```python
from build123d import *

# Parameters (mm, degrees)
BOSS_EXTRUDE1_DEPTH = 26.5
SKETCH3_R           = 10.9
CUT_EXTRUDE1_DEPTH  = 129.322835068
SKETCH6_W           = 26.5
SKETCH6_H           = 26.5
BOSS_EXTRUDE3_DEPTH = 80
SKETCH7_R           = 10.9
CUT_EXTRUDE2_DEPTH  = 200.766738973
FILLET1_R           = 10


with BuildPart() as part:
    # Sketch2 → Boss-Extrude1 (new body)
    with BuildSketch(Plane(origin=(0, 0, 0), x_dir=(1, 0, 0), z_dir=(0, 1, 0))):
        Polygon((0, 0), (0, 66.5), (106.5, 66.5), (106.5, 40), (26.5, 40), (26.5, 0), align=None)
    extrude(amount=BOSS_EXTRUDE1_DEPTH)

    # Sketch3 → Cut-Extrude1 (cut, through all)
    with BuildSketch(Plane.XY):
        with Locations((13.25, 13.25)):
            Circle(SKETCH3_R)
    extrude(amount=-CUT_EXTRUDE1_DEPTH, mode=Mode.SUBTRACT)

    # Sketch6 → Boss-Extrude3 (add)
    with BuildSketch(Plane.ZY):
        with Locations((-53.25, 13.25)):
            Rectangle(SKETCH6_W, SKETCH6_H)
    extrude(amount=BOSS_EXTRUDE3_DEPTH)

    # Sketch7 → Cut-Extrude2 (cut, through all)
    with BuildSketch(Plane.ZY.offset(80)):
        with Locations((-53.25, 13.25)):
            Circle(SKETCH7_R)
    extrude(amount=-CUT_EXTRUDE2_DEPTH, mode=Mode.SUBTRACT)

    # Fillet1
    # the kernel refuses this fillet: 10 mm, written as the material it takes off along each edge
    with BuildSketch(Plane(origin=(106.5, 26.5, -40), x_dir=(0, 0, -1), z_dir=(-1, 0, 0))) as fillet1_piece_1:
        with BuildLine():
            CenterArc((FILLET1_R, FILLET1_R), FILLET1_R, 180, 90)
            Line((0, FILLET1_R), (-FILLET1_R * 0.02, FILLET1_R))
            Line((-FILLET1_R * 0.02, FILLET1_R), (-FILLET1_R * 0.02, -FILLET1_R * 0.02))
            Line((-FILLET1_R * 0.02, -FILLET1_R * 0.02), (FILLET1_R, -FILLET1_R * 0.02))
            Line((FILLET1_R, -FILLET1_R * 0.02), (FILLET1_R, 0))
        make_face()
    extrude(amount=80, mode=Mode.SUBTRACT)
    with BuildSketch(Plane(origin=(106.5, 26.5, -66.5), x_dir=(0, 0, 1), z_dir=(-1, 0, 0)), Plane(origin=(-80, 0, -66.5), x_dir=(0, 0, 1), z_dir=(1, 0, 0))) as fillet1_piece_2:
        with BuildLine():
            CenterArc((FILLET1_R, -FILLET1_R), FILLET1_R, 90, 90)
            Line((0, -FILLET1_R), (-FILLET1_R * 0.02, -FILLET1_R))
            Line((-FILLET1_R * 0.02, -FILLET1_R), (-FILLET1_R * 0.02, FILLET1_R * 0.02))
            Line((-FILLET1_R * 0.02, FILLET1_R * 0.02), (FILLET1_R, FILLET1_R * 0.02))
            Line((FILLET1_R, FILLET1_R * 0.02), (FILLET1_R, 0))
        make_face()
    extrude(amount=186.5, mode=Mode.SUBTRACT)
    with BuildSketch(Plane(origin=(0, 0, 0), x_dir=(0, 1, 0), z_dir=(0, 0, -1)), Plane(origin=(26.5, 26.5, -40), x_dir=(-1, 0, 0), z_dir=(0, 0, 1))) as fillet1_piece_3:
        with BuildLine():
            CenterArc((FILLET1_R, FILLET1_R), FILLET1_R, 180, 90)
            Line((0, FILLET1_R), (-FILLET1_R * 0.02, FILLET1_R))
            Line((-FILLET1_R * 0.02, FILLET1_R), (-FILLET1_R * 0.02, -FILLET1_R * 0.02))
            Line((-FILLET1_R * 0.02, -FILLET1_R * 0.02), (FILLET1_R, -FILLET1_R * 0.02))
            Line((FILLET1_R, -FILLET1_R * 0.02), (FILLET1_R, 0))
        make_face()
    extrude(amount=40, mode=Mode.SUBTRACT)
    with BuildSketch(Plane(origin=(0, 26.5, 0), x_dir=(0, -1, 0), z_dir=(0, 0, -1)), Plane(origin=(26.5, 0, -40), x_dir=(-1, 0, 0), z_dir=(0, 0, 1))) as fillet1_piece_4:
        with BuildLine():
            CenterArc((FILLET1_R, -FILLET1_R), FILLET1_R, 90, 90)
            Line((0, -FILLET1_R), (-FILLET1_R * 0.02, -FILLET1_R))
            Line((-FILLET1_R * 0.02, -FILLET1_R), (-FILLET1_R * 0.02, FILLET1_R * 0.02))
            Line((-FILLET1_R * 0.02, FILLET1_R * 0.02), (FILLET1_R, FILLET1_R * 0.02))
            Line((FILLET1_R, FILLET1_R * 0.02), (FILLET1_R, 0))
        make_face()
    extrude(amount=40, mode=Mode.SUBTRACT)
    with BuildSketch(Plane(origin=(0, 0, -40), x_dir=(0, 0, -1), z_dir=(-1, 0, 0)), Plane(origin=(0, 26.5, -40), x_dir=(0, -1, 0), z_dir=(-1, 0, 0)), Plane(origin=(106.5, 0, -40), x_dir=(0, 0, -1), z_dir=(-1, 0, 0))) as fillet1_piece_5:
        with BuildLine():
            CenterArc((FILLET1_R, -FILLET1_R), FILLET1_R, 90, 90)
            Line((0, -FILLET1_R), (-FILLET1_R * 0.02, -FILLET1_R))
            Line((-FILLET1_R * 0.02, -FILLET1_R), (-FILLET1_R * 0.02, FILLET1_R * 0.02))
            Line((-FILLET1_R * 0.02, FILLET1_R * 0.02), (FILLET1_R, FILLET1_R * 0.02))
            Line((FILLET1_R, FILLET1_R * 0.02), (FILLET1_R, 0))
        make_face()
    extrude(amount=80, mode=Mode.SUBTRACT)
    with BuildSketch(Plane(origin=(106.5, 26.5, -40), x_dir=(0, 0, -1), z_dir=(-1, 0, 0))) as fillet1_piece_6a_section:
        with BuildLine():
            CenterArc((FILLET1_R, FILLET1_R), FILLET1_R, 180, 90)
            Line((0, FILLET1_R), (-FILLET1_R * 0.02, FILLET1_R))
            Line((-FILLET1_R * 0.02, FILLET1_R), (-FILLET1_R * 0.02, -FILLET1_R * 0.02))
            Line((-FILLET1_R * 0.02, -FILLET1_R * 0.02), (FILLET1_R, -FILLET1_R * 0.02))
            Line((FILLET1_R, -FILLET1_R * 0.02), (FILLET1_R, 0))
        make_face()
    fillet1_piece_6a = extrude(amount=105, mode=Mode.PRIVATE)
    fillet1_piece_6a = split(fillet1_piece_6a, bisect_by=Plane(origin=(26.5, 24.236048857, -42.263951143), z_dir=(-1, 0, 0)), keep=Keep.TOP, mode=Mode.PRIVATE)
    with BuildSketch(Plane(origin=(26.5, 26.5, -65), x_dir=(-1, 0, 0), z_dir=(0, 0, 1))) as fillet1_piece_6b_section:
        with BuildLine():
            CenterArc((FILLET1_R, FILLET1_R), FILLET1_R, 180, 90)
            Line((0, FILLET1_R), (-FILLET1_R * 0.02, FILLET1_R))
            Line((-FILLET1_R * 0.02, FILLET1_R), (-FILLET1_R * 0.02, -FILLET1_R * 0.02))
            Line((-FILLET1_R * 0.02, -FILLET1_R * 0.02), (FILLET1_R, -FILLET1_R * 0.02))
            Line((FILLET1_R, -FILLET1_R * 0.02), (FILLET1_R, 0))
        make_face()
    fillet1_piece_6b = extrude(amount=65, mode=Mode.PRIVATE)
    fillet1_piece_6b = split(fillet1_piece_6b, bisect_by=Plane(origin=(24.236048857, 24.236048857, -40), z_dir=(0, 0, -1)), keep=Keep.TOP, mode=Mode.PRIVATE)
    fillet1_piece_6 = fillet1_piece_6a & fillet1_piece_6b
    add(fillet1_piece_6, mode=Mode.SUBTRACT)
    with BuildSketch(Plane(origin=(0, 0, 0), x_dir=(0, 1, 0), z_dir=(0, 0, -1))) as fillet1_piece_7a_section:
        with BuildLine():
            CenterArc((FILLET1_R, FILLET1_R), FILLET1_R, 180, 90)
            Line((0, FILLET1_R), (-FILLET1_R * 0.02, FILLET1_R))
            Line((-FILLET1_R * 0.02, FILLET1_R), (-FILLET1_R * 0.02, -FILLET1_R * 0.02))
            Line((-FILLET1_R * 0.02, -FILLET1_R * 0.02), (FILLET1_R, -FILLET1_R * 0.02))
            Line((FILLET1_R, -FILLET1_R * 0.02), (FILLET1_R, 0))
        make_face()
    fillet1_piece_7a = extrude(amount=65, mode=Mode.PRIVATE)
    fillet1_piece_7a = split(fillet1_piece_7a, bisect_by=Plane(origin=(2.263951143, 2.263951143, -40), z_dir=(0, 0, -1)), keep=Keep.TOP, mode=Mode.PRIVATE)
    with BuildSketch(Plane(origin=(25, 0, -40), x_dir=(0, 0, -1), z_dir=(-1, 0, 0))) as fillet1_piece_7b_section:
        with BuildLine():
            CenterArc((FILLET1_R, -FILLET1_R), FILLET1_R, 90, 90)
            Line((0, -FILLET1_R), (-FILLET1_R * 0.02, -FILLET1_R))
            Line((-FILLET1_R * 0.02, -FILLET1_R), (-FILLET1_R * 0.02, FILLET1_R * 0.02))
            Line((-FILLET1_R * 0.02, FILLET1_R * 0.02), (FILLET1_R, FILLET1_R * 0.02))
            Line((FILLET1_R, FILLET1_R * 0.02), (FILLET1_R, 0))
        make_face()
    fillet1_piece_7b = extrude(amount=105, mode=Mode.PRIVATE)
    fillet1_piece_7b = split(fillet1_piece_7b, bisect_by=Plane(origin=(0, 2.263951143, -42.263951143), z_dir=(1, 0, 0)), keep=Keep.TOP, mode=Mode.PRIVATE)
    fillet1_piece_7 = fillet1_piece_7a & fillet1_piece_7b
    add(fillet1_piece_7, mode=Mode.SUBTRACT)
    with BuildSketch(Plane(origin=(0, 26.5, 0), x_dir=(0, -1, 0), z_dir=(0, 0, -1))) as fillet1_piece_8a_section:
        with BuildLine():
            CenterArc((FILLET1_R, -FILLET1_R), FILLET1_R, 90, 90)
            Line((0, -FILLET1_R), (-FILLET1_R * 0.02, -FILLET1_R))
            Line((-FILLET1_R * 0.02, -FILLET1_R), (-FILLET1_R * 0.02, FILLET1_R * 0.02))
            Line((-FILLET1_R * 0.02, FILLET1_R * 0.02), (FILLET1_R, FILLET1_R * 0.02))
            Line((FILLET1_R, FILLET1_R * 0.02), (FILLET1_R, 0))
        make_face()
    fillet1_piece_8a = extrude(amount=65, mode=Mode.PRIVATE)
    fillet1_piece_8a = split(fillet1_piece_8a, bisect_by=Plane(origin=(2.263951143, 24.236048857, -40), z_dir=(0, 0, -1)), keep=Keep.TOP, mode=Mode.PRIVATE)
    with BuildSketch(Plane(origin=(25, 26.5, -40), x_dir=(0, -1, 0), z_dir=(-1, 0, 0))) as fillet1_piece_8b_section:
        with BuildLine():
            CenterArc((FILLET1_R, -FILLET1_R), FILLET1_R, 90, 90)
            Line((0, -FILLET1_R), (-FILLET1_R * 0.02, -FILLET1_R))
            Line((-FILLET1_R * 0.02, -FILLET1_R), (-FILLET1_R * 0.02, FILLET1_R * 0.02))
            Line((-FILLET1_R * 0.02, FILLET1_R * 0.02), (FILLET1_R, FILLET1_R * 0.02))
            Line((FILLET1_R, FILLET1_R * 0.02), (FILLET1_R, 0))
        make_face()
    fillet1_piece_8b = extrude(amount=105, mode=Mode.PRIVATE)
    fillet1_piece_8b = split(fillet1_piece_8b, bisect_by=Plane(origin=(0, 24.236048857, -42.263951143), z_dir=(1, 0, 0)), keep=Keep.TOP, mode=Mode.PRIVATE)
    fillet1_piece_8 = fillet1_piece_8a & fillet1_piece_8b
    add(fillet1_piece_8, mode=Mode.SUBTRACT)
    with BuildSketch(Plane(origin=(106.5, 0, -40), x_dir=(0, 0, -1), z_dir=(-1, 0, 0))) as fillet1_piece_9a_section:
        with BuildLine():
            CenterArc((FILLET1_R, -FILLET1_R), FILLET1_R, 90, 90)
            Line((0, -FILLET1_R), (-FILLET1_R * 0.02, -FILLET1_R))
            Line((-FILLET1_R * 0.02, -FILLET1_R), (-FILLET1_R * 0.02, FILLET1_R * 0.02))
            Line((-FILLET1_R * 0.02, FILLET1_R * 0.02), (FILLET1_R, FILLET1_R * 0.02))
            Line((FILLET1_R, FILLET1_R * 0.02), (FILLET1_R, 0))
        make_face()
    fillet1_piece_9a = extrude(amount=105, mode=Mode.PRIVATE)
    fillet1_piece_9a = split(fillet1_piece_9a, bisect_by=Plane(origin=(26.5, 2.263951143, -42.263951143), z_dir=(-1, 0, 0)), keep=Keep.TOP, mode=Mode.PRIVATE)
    with BuildSketch(Plane(origin=(26.5, 0, -65), x_dir=(-1, 0, 0), z_dir=(0, 0, 1))) as fillet1_piece_9b_section:
        with BuildLine():
            CenterArc((FILLET1_R, -FILLET1_R), FILLET1_R, 90, 90)
            Line((0, -FILLET1_R), (-FILLET1_R * 0.02, -FILLET1_R))
            Line((-FILLET1_R * 0.02, -FILLET1_R), (-FILLET1_R * 0.02, FILLET1_R * 0.02))
            Line((-FILLET1_R * 0.02, FILLET1_R * 0.02), (FILLET1_R, FILLET1_R * 0.02))
            Line((FILLET1_R, FILLET1_R * 0.02), (FILLET1_R, 0))
        make_face()
    fillet1_piece_9b = extrude(amount=65, mode=Mode.PRIVATE)
    fillet1_piece_9b = split(fillet1_piece_9b, bisect_by=Plane(origin=(24.236048857, 2.263951143, -40), z_dir=(0, 0, -1)), keep=Keep.TOP, mode=Mode.PRIVATE)
    fillet1_piece_9 = fillet1_piece_9a & fillet1_piece_9b
    add(fillet1_piece_9, mode=Mode.SUBTRACT)


solid = part.part
```
The listing builds one solid part. Answer for the finished solid, in the listing's coordinates (mm). A direction names the side the tool comes from. Round coordinates to 2 decimals unless told otherwise and drop trailing zeros. Loops run counter-clockwise (first coordinate to the right, second up) from the corner with the lowest first, then second, coordinate; pieces in that order, holes last. Notation, with made-up numbers: (5, 50) - (41, 50) arc R12 cw to (41, 64) - close; hole circle Ø7 at (14.25, 36.5). An arc over 180 degrees is marked (long way). Use one line per item in the form item = value. Start each with the question number.
1. Consider line 1 (Y direction, x = -18, z = -53.25); line 2 (Z direction, x = 84, y = 13.25). Determine where each line is inside the solid, lowest interval first. Write a range as [from, to].
2. The part is cut by section A-A on y = 13.25. Determine the outline of the cut face in (x, z).
3. For a pull along Y with two mould halves and no side action, classify faces 5 (the face through (0, 13, -20)), 6 (the face through (-34.03, 2.61, -55.61)), 7 (the face through (14, 0, -47)) as pulls with the +Y half, pulls with the -Y half, needs draft (parallel to the pull), parting line crosses it, or undercut.
4. Given pin 1 Ø8 at (y, z) = (20, -16.5) entering from +X; pin 2 Ø2 at (y, z) = (14, -13) entering from -X; pin 3 Ø12 at (x, z) = (37.5, -39) entering from -Y, each flat-ended and moving along its own axis, determine where each tip first touches the part or whether it passes through.
5. The part is cut by section C-C on z = -36.5. Determine the outline of the cut face in (x, y), then the cut area to 3 significant figures.
6. A tool of negligible diameter and unlimited length cuts with its end or side. For faces 1 (the face through (-34.37, 2.85, -43.01)), 2 (the face through (26.5, 13, -20)), 3 (the face through (23.65, 23.49, -19.79)), 4 (the face through (-34.37, 23.49, -42.85)), from which of +Z, -Z, +X, -X, +Y, -Y can it reach the whole face along a straight path? Write none if from no direction.
7. The part is cut by section D-D on z = -48. Determine the outline of the cut face in (x, y).
8. The part is cut by section B-B on x = 89.5. Determine the outline of the cut face in (y, z), then the cut area to 3 significant figures.
Geometry check:
q1.line_1 = [0, 2.35], [24.15, 26.5]
q1.line_2 = [-66.5, -64.15], [-42.35, -40]
q2.outline = (-80, -66.5) - (2.35, -66.5) - (2.35, -64.15) - (-80, -64.15) - close; (-80, -42.35) - (2.35, -42.35) - (2.35, 0) - (0, 0) - (0, -40) - (-80, -40) - close; (24.15, -66.5) - (106.5, -66.5) - (106.5, -64.15) - (24.15, -64.15) - close; (24.15, -42.35) - (106.5, -42.35) - (106.5, -40) - (26.5, -40) - (26.5, 0) - (24.15, 0) - close
q3.face_5 = needs draft
q3.face_6 = undercut
q3.face_7 = pulls with the -Y half
q4.pin_1 = 26.5
q4.pin_2 = 0
q4.pin_3 = 1.34
q5.outline = (0, 10) arc R10 ccw to (10, 0) - (16.5, 0) arc R10 ccw to (26.5, 10) - (26.5, 16.5) arc R10 ccw to (16.5, 26.5) - (10, 26.5) arc R10 ccw to (0, 16.5) - close; hole circle Ø21.8 at (13.25, 13.25)
q5.area = 243 mm^2
q6.face_1 = +Z, -X, -Y
q6.face_2 = +Z, +X, +Y, -Y
q6.face_3 = +Z, +X, +Y
q6.face_4 = +Z, -X, +Y
q7.outline = (-80, 0.2) - (8, 0.2) arc R10 ccw to (10, 0) - (16.5, 0) arc R10 ccw to (18.5, 0.2) - (106.5, 0.2) - (106.5, 3.7) - (18.5, 3.7) arc R10.9 cw to (8, 3.7) - (-80, 3.7) - close; (-80, 22.8) - (8, 22.8) arc R10.9 cw to (18.5, 22.8) - (106.5, 22.8) - (106.5, 26.3) - (18.5, 26.3) arc R10 ccw to (16.5, 26.5) - (10, 26.5) arc R10 ccw to (8, 26.3) - (-80, 26.3) - close
q8.outline = (0, -56.5) arc R10 ccw to (10, -66.5) - (16.5, -66.5) arc R10 ccw to (26.5, -56.5) - (26.5, -50) arc R10 ccw to (16.5, -40) - (10, -40) arc R10 ccw to (0, -50) - close; hole circle Ø21.8 at (13.25, -53.25)
q8.area = 243 mm^2
